Can you work these out from the model? Positions are in its coordinate system, mm. A direction names the side the tool comes from. Coordinates: 2 decimals unless noted, no trailing zeros. Order: outer loops, then holes, each group sorted by start corner. A loop starts at its lowest first (then second) coordinate and runs counter-clockwise, first axis right, second up. Notation, with made-up numbers: M 67,42 L 87,42 A28 cw 87,71 Z; hole C 47,49.5 d10. An arc over 180 degrees is marked long. Answer as a JSON object with one key per item and string values.
from build123d import *

# Parameters (mm, degrees)
SKETCH1_R           = 38.1
SKETCH1_R_2         = 3.175
BOSS_EXTRUDE1_DEPTH = 19.05
SKETCH2_R           = 38.1
SKETCH2_R_2         = 28.575
BOSS_EXTRUDE2_DEPTH = 3.175
BOSS_EXTRUDE3_START = 3.175
SKETCH3_R           = 38.1
SKETCH3_R_2         = 28.575
BOSS_EXTRUDE3_DEPTH = 3.175
SKETCH4_R           = 12.7
SKETCH4_R_2         = 3.175
BOSS_EXTRUDE4_DEPTH = 3.175
BOSS_EXTRUDE5_START = 3.175
SKETCH5_R           = 12.7
SKETCH5_R_2         = 3.175
BOSS_EXTRUDE5_DEPTH = 3.175
FILLET1_R           = 3.175


with BuildPart() as part:
    # Sketch1 → Boss-Extrude1 (new body)
    with BuildSketch(Plane(origin=(0, 0, 0), x_dir=(1, 0, 0), z_dir=(0, 1, 0))):
        with Locations(Location((0, 0, 0), (0, 0, 90))):
            Circle(SKETCH1_R)
        with Locations(Location((0, 0, 0), (0, 0, 90))):
            Circle(SKETCH1_R_2, mode=Mode.SUBTRACT)
    extrude(amount=BOSS_EXTRUDE1_DEPTH)

    # Sketch2 → Boss-Extrude2 (add)
    with BuildSketch(Plane(origin=(0, 19.05, 0), x_dir=(1, 0, 0), z_dir=(0, 1, 0))):
        with Locations(Location((0, 0, 0), (0, 0, 90))):
            Circle(SKETCH2_R)
        with Locations(Location((0, 0, 0), (0, 0, 270))):
            Circle(SKETCH2_R_2, mode=Mode.SUBTRACT)
    extrude(amount=BOSS_EXTRUDE2_DEPTH)

    # Sketch3 → Boss-Extrude3 (add)
    with BuildSketch(Plane.XZ.offset(BOSS_EXTRUDE3_START)):
        with Locations(Location((0, 0, 0), (0, 0, 270))):
            Circle(SKETCH3_R)
        with Locations(Location((0, 0, 0), (0, 0, 90))):
            Circle(SKETCH3_R_2, mode=Mode.SUBTRACT)
    extrude(amount=-BOSS_EXTRUDE3_DEPTH)

    # Sketch4 → Boss-Extrude4 (add)
    with BuildSketch(Plane(origin=(0, 19.05, 0), x_dir=(1, 0, 0), z_dir=(0, 1, 0))):
        with Locations(Location((0, 0, 0), (0, 0, 270))):
            Circle(SKETCH4_R)
        with Locations(Location((0, 0, 0), (0, 0, 90))):
            Circle(SKETCH4_R_2, mode=Mode.SUBTRACT)
    extrude(amount=BOSS_EXTRUDE4_DEPTH)

    # Sketch5 → Boss-Extrude5 (add)
    with BuildSketch(Plane.XZ.offset(BOSS_EXTRUDE5_START)):
        with Locations(Location((0, 0, 0), (0, 0, 90))):
            Circle(SKETCH5_R)
        with Locations(Location((0, 0, 0), (0, 0, 270))):
            Circle(SKETCH5_R_2, mode=Mode.SUBTRACT)
    extrude(amount=-BOSS_EXTRUDE5_DEPTH)

    # Fillet1
    fillet1_edges = [part.edges().sort_by_distance(p)[0] for p in [
        (0, 0, -28.575),
        (0, 19.05, -12.7),
        (0, 0, -12.7),
        (0, 19.05, -28.575),
    ]]
    fillet(fillet1_edges, radius=FILLET1_R - 0.0001)  # a hair under: the kernel refuses the full size


solid = part.part
Item 1: I want a section at D-D, the plane x = 29.5. Write out the boundary of the cut face in (y, z) (3 decimals).
Answers follow:
{"outline": "M -3.175,-24.111 L 22.225,-24.111 L 22.225,24.111 L -3.175,24.111 Z"}
Item 2: Which directions (+Z, -Z, +X, -X, +Y, -Y) give clear straight access to the entire face, cutting with the end or side of a thin tool? Please do faces 1 (the flat face through (3, -3.175, 3)), 2 (the flat face through (11, 0, 12)).
Answers follow:
{"face 1": "+Z, -Z, +X, -X, -Y", "face 2": "-Y"}
Item 3: I want a section at C-C, the plane y = 17. Write out the boundary of the cut face in (x, z) (3 decimals).
Answers follow:
{"outline": "C 0,0 d76.2; hole C 0,0 d6.35"}
Item 4: I'm going to push flat-ended pins straight in: pin 1 (8 mm diameter, centred on x = 15, y = 6, fed in from +Z); pin 2 (4 mm diameter, centred on y = 15.5, z = 2.5, fed in from +X); pin 3 (4 mm diameter, centred on x = 0, z = 0, fed in from +Y); pin 4 (10 mm diameter, centred on y = 10.5, z = -9.5, fed in from +X). Where does each tip first touch, or does it pass through?
Answers follow:
{"pin 1": "stops at z = 36.48", "pin 2": "stops at x = 38.1", "pin 3": "passes through", "pin 4": "stops at x = 37.83"}
Item 5: If we mould it in two halves opening along Z, with no side actions, what happens to faces 3 (the flat face through (11, 19.05, 12)), 4 (the flat face through (28.4, -3.175, -5.5)), 5 (the cylindrical face through (-23.183, 9.347, 30.235))? For each: pulls with the +Z half, pulls with the -Z half, needs draft (parallel to the pull), parting line crosses it, or undercut.
Answers follow:
{"face 3": "undercut", "face 4": "needs draft", "face 5": "parting line crosses it"}
Item 6: Please list where these lines run through material, in increasing order: line 1 (Y direction, x = -0.5, z = -19.5); line 2 (X direction, y = 20, z = 14.5); line 3 (Z direction, x = 0, y = 14) (3 decimals).
Answers follow:
{"line 1": "y = 0 to 19.05", "line 2": "x = -35.23 to -23.56, 23.56 to 35.23", "line 3": "z = -38.1 to -3.175, 3.175 to 38.1"}
